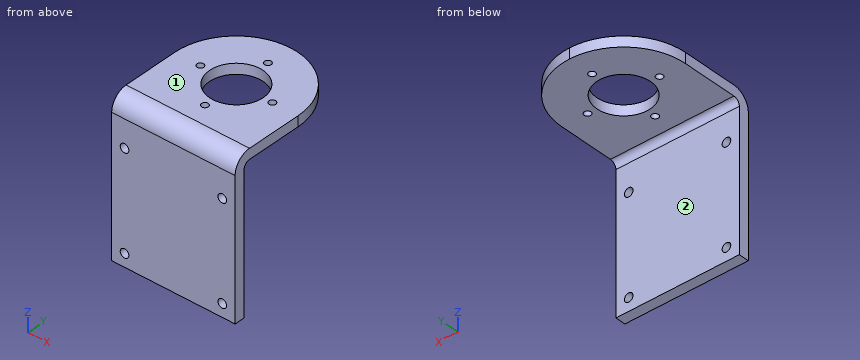
```python
from build123d import *

# Parameters (mm, degrees)
SKETCH_10_W                      = 60
SKETCH_10_H                      = 60
SM_BASE_FLANGE_2_DEPTH           = 5
SM_EDGE_FLANGE_2_STRIP_W         = 26
SM_EDGE_FLANGE_2_STRIP_H         = 5
SM_EDGE_FLANGE_2_STRIP_CUT_DEPTH = 60
SM_EDGE_FLANGE_2_DEPTH           = 60
SKETCH_19_R                      = 1.65
SKETCH_19_R_2                    = 13
CUT_EXTRUDE_2_DEPTH              = 5
CUT_EXTRUDE_START                = -30
SKETCH_28_R                      = 2.1
CUT_EXTRUDE_4_DEPTH              = 5
CUT_EXTRUDE_5_DEPTH              = 5


# Sheet-metal steps are written as plain solids
with BuildPart() as part:
    # 草图10 → 基体-法兰2 (new body)
    with BuildSketch(Plane.XY):
        Rectangle(SKETCH_10_W, SKETCH_10_H)
    extrude(amount=-SM_BASE_FLANGE_2_DEPTH)

    # 边线-法兰2 strip (across the edge) → 边线-法兰2 strip cut (cut)
    with BuildSketch(Plane(origin=(30, -30, -5), x_dir=(0, 1, 0), z_dir=(-1, 0, 0))):
        with Locations((-10, -2.5)):
            Rectangle(SM_EDGE_FLANGE_2_STRIP_W, SM_EDGE_FLANGE_2_STRIP_H)
    extrude(amount=SM_EDGE_FLANGE_2_STRIP_CUT_DEPTH, mode=Mode.SUBTRACT)

    # 边线-法兰2 section (across the edge) → 边线-法兰2 (add)
    with BuildSketch(Plane(origin=(30, -30, -5), x_dir=(0, 1, 0), z_dir=(-1, 0, 0))):
        with BuildLine():
            Line((-5, 3), (-5, 70))
            Line((-5, 70), (0, 70))
            Line((0, 70), (0, 3))
            ThreePointArc((0, 3), (0.878679656, 0.878679656), (3, 0))
            Line((3, 0), (3, -5))
            ThreePointArc((3, -5), (-2.656854249, -2.656854249), (-5, 3))
        make_face()
    extrude(amount=SM_EDGE_FLANGE_2_DEPTH)

    # 草图19 → 切除-拉伸2 (cut)
    with BuildSketch(Plane.XY):
        with Locations(Location((-17.5, 0, 0), (0, 0, 180))):
            Circle(SKETCH_19_R)
        with Locations(Location((17.5, 0, 0), (0, 0, 180))):
            Circle(SKETCH_19_R)
        with Locations(Location((0, 17.5, 0), (0, 0, 180))):
            Circle(SKETCH_19_R)
        with Locations(Location((0, -17.5, 0), (0, 0, 180))):
            Circle(SKETCH_19_R)
        with Locations(Location((0, 0, 0), (0, 0, 180))):
            Circle(SKETCH_19_R_2)
    extrude(amount=-CUT_EXTRUDE_2_DEPTH, mode=Mode.SUBTRACT)

    # 草图28 → 切除-拉伸4 (cut)
    with BuildSketch(Plane(origin=(0, 0, 0), x_dir=(1, 0, 0), z_dir=(0, 1, 0)).offset(CUT_EXTRUDE_START)):
        with Locations(Location((-23.75, 21.25, 0), (0, 0, 270))):
            Circle(SKETCH_28_R)
        with Locations(Location((-23.75, 68.75, 0), (0, 0, 270))):
            Circle(SKETCH_28_R)
        with Locations(Location((23.75, 68.75, 0), (0, 0, 270))):
            Circle(SKETCH_28_R)
        with Locations(Location((23.75, 21.25, 0), (0, 0, 270))):
            Circle(SKETCH_28_R)
    extrude(amount=-CUT_EXTRUDE_4_DEPTH, mode=Mode.SUBTRACT)

    # 草图29 → 切除-拉伸5 (cut)
    with BuildSketch(Plane.XY):
        with BuildLine():
            ThreePointArc((-30, 0), (-21.213203436, 21.213203436), (0, 30))
            Line((0, 30), (-30, 30))
            Line((-30, 30), (-30, 0))
        make_face()
        with BuildLine():
            Line((30, 30), (0, 30))
            ThreePointArc((0, 30), (21.213203436, 21.213203436), (30, 0))
            Line((30, 0), (30, 30))
        make_face()
    extrude(amount=-CUT_EXTRUDE_5_DEPTH, mode=Mode.SUBTRACT)


solid = part.part
```
Verification items for the finished model (mm, model axes). Face numbers are marked on the shaded views. A direction names the side the tool comes from. Round coordinates to 2 decimals unless told otherwise and drop trailing zeros. Write each loop counter-clockwise with the first axis right and the second up, starting at its lowest first coordinate (ties: lowest second). Pieces come first, ordered by that corner, then holes.
1. Section check C-C on x = -5.5. Enter the section's corners in (y, z).
2. Section check D-D on x = -23.75. Enter the section's corners in (y, z).
3. Section check B-B on z = -68.75. Enter the section's corners in (x, y).
4. Scan lines: L1, parallel to X at y = -32.55, z = -21.25; L2, parallel to Y at x = 0, z = -3 (3 decimals); L3, parallel to Y at x = -17, z = -52.5. Record each from-to range of solid material in increasing order.
5. Gauge pin test, flat ends, axial feed: P1, Ø17, axis at x = 12, y = 2.5, coming from the -Z side; P2, Ø5, axis at x = 23.75, z = -68.75, coming from the +Y side; P3, Ø4, axis at x = 23.75, z = -21.25, coming from the -Y side. Record the tip position at first contact, or that the pin passes through.
6. Access from +Z, -Z, +X, -X, +Y, -Y to the whole of each face (thin tool, end or side, straight path). Record for the marked faces 1 and 2.
7. Section check A-A on y = -17.5. Enter the section's corners in (x, z), plus the area to 4 significant figures.
Answer:
1. outline: (-35, -75) - (-30, -75) - (-30, -8) arc R3 cw to (-27, -5) - (-11.78, -5) - (-11.78, 0) - (-27, 0) arc R8 ccw to (-35, -8) - close; (11.78, -5) - (29.49, -5) - (29.49, 0) - (11.78, 0) - close
2. outline: (-35, -75) - (-30, -75) - (-30, -70.85) - (-35, -70.85) - close; (-35, -66.65) - (-30, -66.65) - (-30, -23.35) - (-35, -23.35) - close; (-35, -19.15) - (-30, -19.15) - (-30, -8) arc R3 cw to (-27, -5) - (18.33, -5) - (18.33, 0) - (-27, 0) arc R8 ccw to (-35, -8) - close
3. outline: (-30, -35) - (-25.85, -35) - (-25.85, -30) - (-30, -30) - close; (-21.65, -35) - (21.65, -35) - (21.65, -30) - (-21.65, -30) - close; (25.85, -35) - (30, -35) - (30, -30) - (25.85, -30) - close
4. L1: x = -30 to -25.85, -21.65 to 21.65, 25.85 to 30
4. L2: y = -33.245 to -19.15, -15.85 to -13, 13 to 15.85, 19.15 to 30
4. L3: y = -35 to -30
5. P1: stops at z = -5
5. P2: stops at y = -30
5. P3: passes through
6. face 1: +Z, +X, -X, +Y, -Y
6. face 2: -Z, +X, -X, +Y
7. outline: (-30, -5) - (-1.65, -5) - (-1.65, 0) - (-30, 0) - close; (1.65, -5) - (30, -5) - (30, 0) - (1.65, 0) - close
7. area: 283.5 mm2
